```python
from build123d import *

# Parameters (mm, degrees)
SZKIC2_R                              = 30
SZKIC2_R_2                            = 27
DODANIE_WYCI_GNI_CIE4_DEPTH           = 200
OTWORY_USTALAJ_CE_10_0MM1_D           = 10
OTWORY_USTALAJ_CE_10_0MM1_CSINK_D     = 10.05
OTWORY_USTALAJ_CE_10_0MM1_CSINK_ANGLE = 90


with BuildPart() as part:
    # Szkic2 → Dodanie-wyciągnięcie4 (new body)
    with BuildSketch(Plane.XY):
        Circle(SZKIC2_R)
        Circle(SZKIC2_R_2, mode=Mode.SUBTRACT)
    extrude(amount=DODANIE_WYCI_GNI_CIE4_DEPTH)

    # Otwory ustalające Ø10.0mm1 (through all)
    with Locations(Plane(origin=(30, 0, 50), x_dir=(0, 1, 0), z_dir=(1, 0, 0))):
        with Locations((0, 0)):
            CounterSinkHole(OTWORY_USTALAJ_CE_10_0MM1_D / 2, OTWORY_USTALAJ_CE_10_0MM1_CSINK_D / 2, counter_sink_angle=OTWORY_USTALAJ_CE_10_0MM1_CSINK_ANGLE)


solid = part.part
```
Check sheet for the modelled part. Datum: model origin and axes. Units: mm. Round coordinates to 2 decimals unless told otherwise and drop trailing zeros. Loops run counter-clockwise (first coordinate to the right, second up) from the corner with the lowest first, then second, coordinate; pieces in that order, holes last. Notation, with made-up numbers: (69, -2.75) -> (75, -2.75) arc R25 cw to (75, 25.25) -> close; hole circle Ø10 at (-37.5, 39). An arc over 180 degrees is marked (long way). Write item = value, one per line. Start each with the question number.
1) Sectioned sample at A-A, the plane x = 0. Record the cut outline in (y, z).
2) Sectioned sample at B-B, the plane z = 50. Record the cut outline in (x, y).
3) Sectioned sample at C-C, the plane z = 17. Record the cut outline in (x, y).
4) Gauge pin test, flat ends, axial feed: pin 1 Ø3 at (y, z) = (-14.5, 36.5) entering from +X; pin 2 Ø10 at (x, z) = (-21, 168) entering from +Y; pin 3 Ø2 at (x, z) = (10, 121.5) entering from -Y. Record the tip position at first contact, or that the pin passes through.
5) Thickness scan on probe 1 along X at (y, z) = (-1.5, 26); probe 2 along Y at (x, z) = (0, 120); probe 3 along X at (y, z) = (22, 154). Record the ranges inside material, lowest first.
6) Release check for a two-part mould opening along Y. For faces 1 (the flat face through (-25, 11, 200)), 2 (the cylindrical face through (27.712, -11.49, 98.6)), 3 (the cylindrical face through (28, -3, 54)) record: released by +Y, released by -Y, zero draft, split by the parting line, or undercut.
Results are:
q1.outline = (-30, 0) -> (-27, 0) -> (-27, 200) -> (-30, 200) -> close; (27, 0) -> (30, 0) -> (30, 200) -> (27, 200) -> close
q2.outline = (-29.58, -5) arc R30 ccw to (29.58, -5) -> (26.53, -5) arc R27 cw to (-26.53, -5) -> close; (-29.58, 5) -> (-26.53, 5) arc R27 cw to (26.53, 5) -> (29.58, 5) arc R30 ccw to start
q3.outline = circle Ø60 at (0, 0); hole circle Ø54 at (0, 0)
q4.pin_1 = 27.04
q4.pin_2 = 25.38
q4.pin_3 = -28.62
q5.probe_1 = -29.96 to -26.96, 26.96 to 29.96
q5.probe_2 = -30 to -27, 27 to 30
q5.probe_3 = -20.4 to -15.65, 15.65 to 20.4
q6.face_1 = zero draft
q6.face_2 = split by the parting line
q6.face_3 = undercut
